```python
from build123d import *

# Parameters (mm, degrees)
EXTRUDE_1_DEPTH           = 10
FILLET_1_R                = 6
SKETCH_2_W                = 40.5
SKETCH_2_H                = 22
CUT_EXTRUDE_1_DEPTH       = 11
HOLE_WIZARD_4_0_1_D       = 4
HOLE_WIZARD_4_0_1_DEPTH   = 6
HOLE_WIZARD_4_0_1_TIP     = 1.201721238
HOLE_WIZARD_7_0_7_1_D     = 7
HOLE_WIZARD_7_0_7_1_DEPTH = 6
HOLE_WIZARD_7_0_7_1_TIP   = 2.103012167
HOLE_WIZARD_M41_D         = 4.3
CUT_EXTRUDE_4_DEPTH       = 4.5
HOLE_WIZARD_M42_D         = 4.3
CUT_EXTRUDE_7_DEPTH       = 3.2
SKETCH_19_W               = 4.5
SKETCH_19_H               = 4.156921938
CUT_EXTRUDE_13_DEPTH      = 0.15
SKETCH_21_W               = 4.5
SKETCH_21_H               = 4.156921938
CUT_EXTRUDE_14_DEPTH      = 0.15
SKETCH_22_W               = 4.5
SKETCH_22_H               = 4.156921938
CUT_EXTRUDE_15_DEPTH      = 0.15
SKETCH_23_W               = 4.5
SKETCH_23_H               = 4.156921938
CUT_EXTRUDE_16_DEPTH      = 0.15
CUT_EXTRUDE_17_DEPTH      = 4
HOLE_WIZARD_M2_21_D       = 2
HOLE_WIZARD_M2_21_DEPTH   = 10
HOLE_WIZARD_M2_21_TIP     = 0.600860619
CUT_EXTRUDE_19_DEPTH      = 0.375
CUT_EXTRUDE_20_DEPTH      = 0.375


with BuildPart() as part:
    # Эскиз1 → Бобышка-Вытянуть1 (new body)
    with BuildSketch(Plane.XY):
        Polygon((0, 0), (64, 0), (64, 34.019237886), (49, 60), (15, 60), (0, 34.02), align=None)
    extrude(amount=EXTRUDE_1_DEPTH)

    # Скругление1
    fillet_1_edges = [part.edges().sort_by_distance(p)[0] for p in [
        (0, 34.02, 5),
        (15, 60, 5),
        (49, 60, 5),
        (64, 34.019237886, 5),
        (64, 0, 5),
        (0, 0, 5),
    ]]
    fillet(fillet_1_edges, radius=FILLET_1_R)

    # Эскиз2 → Вырез-Вытянуть1 (cut, through all)
    with BuildSketch(Plane.XY.offset(10)):
        with Locations((32, 21)):
            Rectangle(SKETCH_2_W, SKETCH_2_H)
    extrude(amount=-CUT_EXTRUDE_1_DEPTH, mode=Mode.SUBTRACT)

    # Отверстия под штифты Ø4.0 мм1
    with Locations(Plane.XY.offset(10)):
        with Locations((27.499949191, 55), (36.5, 55)):
            Hole(HOLE_WIZARD_4_0_1_D / 2, depth=HOLE_WIZARD_4_0_1_DEPTH)
            with Locations((0, 0, -(HOLE_WIZARD_4_0_1_DEPTH + HOLE_WIZARD_4_0_1_TIP / 2))):  # 118° drill point
                Cone(0, HOLE_WIZARD_4_0_1_D / 2, HOLE_WIZARD_4_0_1_TIP, mode=Mode.SUBTRACT)

    # Диаметр отверстия Ø7.0 (7)1
    with Locations(Plane.XY.offset(10)):
        with Locations((19.949949191, 39), (44.05, 39)):
            Hole(HOLE_WIZARD_7_0_7_1_D / 2, depth=HOLE_WIZARD_7_0_7_1_DEPTH)
            with Locations((0, 0, -(HOLE_WIZARD_7_0_7_1_DEPTH + HOLE_WIZARD_7_0_7_1_TIP / 2))):  # 118° drill point
                Cone(0, HOLE_WIZARD_7_0_7_1_D / 2, HOLE_WIZARD_7_0_7_1_TIP, mode=Mode.SUBTRACT)

    # Сверло под метчик  спиральное M41 (through all)
    with Locations(Plane.XY.offset(10)):
        with Locations((56, 26), (56, 16), (8, 26), (8, 16)):
            Hole(HOLE_WIZARD_M41_D / 2)

    # Эскиз9 → Вырез-Вытянуть4 (cut)
    with BuildSketch(Plane(origin=(0, 0, 10), x_dir=(-1, 0, 0), z_dir=(0, 0, -1))):
        Polygon((-56, 30.156921938), (-59.6, 28.078460969), (-59.6, 23.921539031), (-56, 21.843078062), (-52.4, 23.921539031), (-52.4, 28.078460969), align=None)
        Polygon((-56, 20.156921938), (-59.6, 18.078460969), (-59.6, 13.921539031), (-56, 11.843078062), (-52.4, 13.921539031), (-52.4, 18.078460969), align=None)
        Polygon((-8, 30.156921938), (-11.6, 28.078460969), (-11.6, 23.921539031), (-8, 21.843078062), (-4.4, 23.921539031), (-4.4, 28.078460969), align=None)
        Polygon((-8, 20.156921938), (-11.6, 18.078460969), (-11.6, 13.921539031), (-8, 11.843078062), (-4.4, 13.921539031), (-4.4, 18.078460969), align=None)
    extrude(amount=CUT_EXTRUDE_4_DEPTH, mode=Mode.SUBTRACT)

    # Сверло под метчик  спиральное M42 (through all)
    with Locations(Plane.XY.offset(10)):
        with Locations((32, 49), (6, 6), (58, 6)):
            Hole(HOLE_WIZARD_M42_D / 2)

    # Эскиз18 → Вырез-Вытянуть7 (cut)
    with BuildSketch(Plane(origin=(0, 0, 0), x_dir=(-1, 0, 0), z_dir=(0, 0, -1))):
        Polygon((-32, 53.156921938), (-35.6, 51.078460969), (-35.6, 46.921539031), (-32, 44.843078062), (-28.4, 46.921539031), (-28.4, 51.078460969), align=None)
        Polygon((-58, 10.156921938), (-61.6, 8.078460969), (-61.6, 3.921539031), (-58, 1.843078062), (-54.4, 3.921539031), (-54.4, 8.078460969), align=None)
        Polygon((-6, 10.156921938), (-9.6, 8.078460969), (-9.6, 3.921539031), (-6, 1.843078062), (-2.4, 3.921539031), (-2.4, 8.078460969), align=None)
    extrude(amount=-CUT_EXTRUDE_7_DEPTH, mode=Mode.SUBTRACT)

    # Эскиз19 → Вырез-Вытянуть13 (cut)
    with BuildSketch(Plane.ZY.offset(-52.25)):
        with Locations((7.75, 26)):
            Rectangle(SKETCH_19_W, SKETCH_19_H)
    extrude(amount=-CUT_EXTRUDE_13_DEPTH, mode=Mode.SUBTRACT)

    # Эскиз21 → Вырез-Вытянуть14 (cut)
    with BuildSketch(Plane(origin=(11.75, 0, 0), x_dir=(0, 0, -1), z_dir=(1, 0, 0))):
        with Locations((-7.75, 26)):
            Rectangle(SKETCH_21_W, SKETCH_21_H)
    extrude(amount=-CUT_EXTRUDE_14_DEPTH, mode=Mode.SUBTRACT)

    # Эскиз22 → Вырез-Вытянуть15 (cut)
    with BuildSketch(Plane.ZY.offset(-52.25)):
        with Locations((7.75, 16)):
            Rectangle(SKETCH_22_W, SKETCH_22_H)
    extrude(amount=-CUT_EXTRUDE_15_DEPTH, mode=Mode.SUBTRACT)

    # Эскиз23 → Вырез-Вытянуть16 (cut)
    with BuildSketch(Plane(origin=(11.75, 0, 0), x_dir=(0, 0, -1), z_dir=(1, 0, 0))):
        with Locations((-7.75, 16)):
            Rectangle(SKETCH_23_W, SKETCH_23_H)
    extrude(amount=-CUT_EXTRUDE_16_DEPTH, mode=Mode.SUBTRACT)

    # Эскиз12 → Вырез-Вытянуть17 (cut)
    with BuildSketch(Plane(origin=(0, 10, 0), x_dir=(1, 0, 0), z_dir=(0, 1, 0))):
        Polygon((34.309375673, -8), (33.154675134, -6), (30.845274057, -6), (29.690573519, -8), (30.845274057, -10), (33.154675134, -10), align=None)
    extrude(amount=-CUT_EXTRUDE_17_DEPTH, mode=Mode.SUBTRACT)

    # Сверло под метчик  спиральное M2.21
    with Locations(Plane(origin=(0, 0, 0), x_dir=(-1, 0, 0), z_dir=(0, -1, 0))):
        with Locations((-32, -8)):
            Hole(HOLE_WIZARD_M2_21_D / 2, depth=HOLE_WIZARD_M2_21_DEPTH)
            with Locations((0, 0, -(HOLE_WIZARD_M2_21_DEPTH + HOLE_WIZARD_M2_21_TIP / 2))):  # 118° drill point
                Cone(0, HOLE_WIZARD_M2_21_D / 2, HOLE_WIZARD_M2_21_TIP, mode=Mode.SUBTRACT)

    # Эскиз29 → Вырез-Вытянуть19 (cut, symmetric)
    with BuildSketch(Plane(origin=(0, 21, 0), x_dir=(1, 0, 0), z_dir=(0, 1, 0))):
        Polygon((5.75, 0), (12.75, 0), (12.75, -0.612420645), align=None)
    extrude(amount=CUT_EXTRUDE_19_DEPTH, both=True, mode=Mode.SUBTRACT)

    # Эскиз29<3> → Вырез-Вытянуть20 (cut, symmetric)
    with BuildSketch(Plane(origin=(0, 21, 0), x_dir=(1, 0, 0), z_dir=(0, 1, 0))):
        Polygon((51.25, 0), (51.25, -0.612420645), (58.25, 0), align=None)
    extrude(amount=CUT_EXTRUDE_20_DEPTH, both=True, mode=Mode.SUBTRACT)


solid = part.part
```
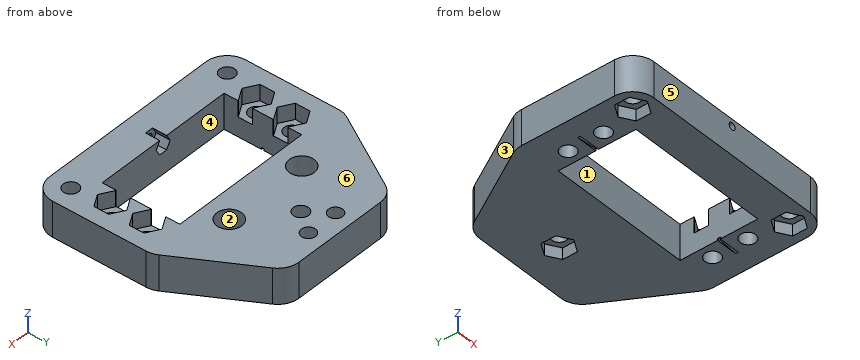
Geometry: final body of the model. Coordinates: model frame, mm. Face numbers are marked on the shaded views. A direction names the side the tool comes from. Round coordinates to 2 decimals unless told otherwise and drop trailing zeros. Write each loop counter-clockwise with the first axis right and the second up, starting at its lowest first coordinate (ties: lowest second). Pieces come first, ordered by that corner, then holes. Notation, with made-up numbers: M -5,49 L -1,49 A14 cw -1,67 Z; hole C -36.75,-9.75 d9. An arc over 180 degrees is marked long. Answer in a Markdown table with one row per item. Add a question column.
(1) Ray query, L1, parallel to Y at x = 23.5, z = 7.5; L2, parallel to Y at x = 23, z = 8.75; L3, parallel to Y at x = 31.5, z = 1.25. Return the intervals inside material, ascending.
(2) Reachability of the marked faces 1, 2 and 3 from +Z, -Z, +X, -X, +Y, -Y: full face, straight path, thin tool, end or side. Return the list, or none.
(3) Cut plane B-B, the plane y = 16. Return the cut outline in (x, z), then the cut area to 3 significant figures.
(4) Draft query along Y for the marked faces 4, 5 and 6. Return one class per face: pulls with the +Y half, pulls with the -Y half, needs draft (parallel to the pull), parting line crosses it, or undercut.
(5) Cut plane A-A, the plane y = 5. Return the cut outline in (x, z).
(6) Contact query for flat-ended pins moving along their axis: pin 1 (5 mm diameter, centred on x = 6, y = 6, fed in from -Z); pin 2 (5.5 mm diameter, centred on x = 32, y = 49, fed in from +Z); pin 3 (1.8 mm diameter, centred on x = 32, y = 9, fed in from +Z); pin 4 (1.2 mm diameter, centred on x = 32, z = 8, fed in from -Y). Output: stop coordinate, or through.
(7) Cut plane D-D, the plane y = 49. Return the cut outline in (x, z), then the cut area to 3 significant figures.
(8) Cut plane C-C, the plane x = 49. Return the cut outline in (y, z), then the cut area to 3 significant figures.
Established:
| question | item | result |
|---|---|---|
| 1 | L1 | 0 to 10, 32 to 60 |
| 1 | L2 | 0 to 10, 32 to 37.28, 40.72 to 60 |
| 1 | L3 | 0 to 10, 32 to 45.13, 52.87 to 60 |
| 2 | face 1 | +Z, -Z |
| 2 | face 2 | +Z |
| 2 | face 3 | +Z, -Z, -X, +Y |
| 3 | outline | M 0,0 L 5.85,0 L 5.85,5.5 L 4.4,5.5 L 4.4,10 L 0,10 Z; M 10.15,0 L 11.75,0 L 11.75,5.5 L 10.15,5.5 Z; M 52.25,0 L 53.85,0 L 53.85,5.5 L 52.25,5.5 Z; M 58.15,0 L 64,0 L 64,10 L 59.6,10 L 59.6,5.5 L 58.15,5.5 Z |
| 3 | area | 122 mm² |
| 4 | face 4 | undercut |
| 4 | face 5 | pulls with the -Y half |
| 4 | face 6 | needs draft |
| 5 | outline | M 0.08,0 L 2.4,0 L 2.4,3.2 L 4.1,3.2 L 4.1,10 L 0.08,10 Z; M 7.9,3.2 L 9.6,3.2 L 9.6,0 L 54.4,0 L 54.4,3.2 L 56.1,3.2 L 56.1,10 L 7.9,10 Z; M 59.9,3.2 L 61.6,3.2 L 61.6,0 L 63.92,0 L 63.92,10 L 59.9,10 Z; hole C 32,8 d2 |
| 6 | pin 1 | z = 3.2 |
| 6 | pin 2 | z = 10 |
| 6 | pin 3 | z = 6 |
| 6 | pin 4 | y = 32 |
| 7 | outline | M 8.65,0 L 28.4,0 L 28.4,3.2 L 29.85,3.2 L 29.85,10 L 8.65,10 Z; M 34.15,3.2 L 35.6,3.2 L 35.6,0 L 55.35,0 L 55.35,10 L 34.15,10 Z |
| 7 | area | 415 mm² |
| 8 | outline | M 0,0 L 10,0 L 10,10 L 0,10 Z; M 32,0 L 58.9,0 L 58.9,10 L 32,10 Z |
| 8 | area | 369 mm² |
